from build123d import *

# Parameters (mm, degrees)
ESTRUSIONE_ESTRUSIONE1_DEPTH = 10
FORI_FILETTATI_5_0MM1_D      = 5
FORI_FILETTATI_5_0MM1_DEPTH  = 10
FORI_FILETTATI_5_0MM1_TIP    = 1.502151548
FORI_FILETTATI_5_0MM2_D      = 5
FORI_FILETTATI_5_0MM2_DEPTH  = 10
FORI_FILETTATI_5_0MM2_TIP    = 1.502151548


with BuildPart() as part:
    # Schizzo2 → Estrusione-Estrusione1 (new body)
    with BuildSketch(Plane(origin=(0, 0, 0), x_dir=(0, 0, -1), z_dir=(1, 0, 0))):
        with BuildLine():
            Line((-28, -7), (-9, -7))
            Line((-9, -7), (-9, 0))
            ThreePointArc((-9, 0), (0, 9), (9, 0))
            Line((9, 0), (9, -7))
            Line((9, -7), (28, -7))
            Line((28, -7), (28, -8))
            Line((28, -8), (8, -8))
            Line((8, -8), (8, 0))
            ThreePointArc((8, 0), (0, 8), (-8, 0))
            Line((-8, 0), (-8, -8))
            Line((-8, -8), (-28, -8))
            Line((-28, -8), (-28, -7))
        make_face()
    extrude(amount=ESTRUSIONE_ESTRUSIONE1_DEPTH)

    # Fori filettati Ø5.0mm1
    with Locations(Plane(origin=(5, -7, -18), x_dir=(0, 0, 1), z_dir=(0, 1, 0))):
        with Locations((0, 0)):
            Hole(FORI_FILETTATI_5_0MM1_D / 2, depth=FORI_FILETTATI_5_0MM1_DEPTH)
            with Locations((0, 0, -(FORI_FILETTATI_5_0MM1_DEPTH + FORI_FILETTATI_5_0MM1_TIP / 2))):  # 118° drill point
                Cone(0, FORI_FILETTATI_5_0MM1_D / 2, FORI_FILETTATI_5_0MM1_TIP, mode=Mode.SUBTRACT)

    # Fori filettati Ø5.0mm2
    with Locations(Plane(origin=(5, -7, 18), x_dir=(0, 0, 1), z_dir=(0, 1, 0))):
        with Locations((0, 0)):
            Hole(FORI_FILETTATI_5_0MM2_D / 2, depth=FORI_FILETTATI_5_0MM2_DEPTH)
            with Locations((0, 0, -(FORI_FILETTATI_5_0MM2_DEPTH + FORI_FILETTATI_5_0MM2_TIP / 2))):  # 118° drill point
                Cone(0, FORI_FILETTATI_5_0MM2_D / 2, FORI_FILETTATI_5_0MM2_TIP, mode=Mode.SUBTRACT)


solid = part.part
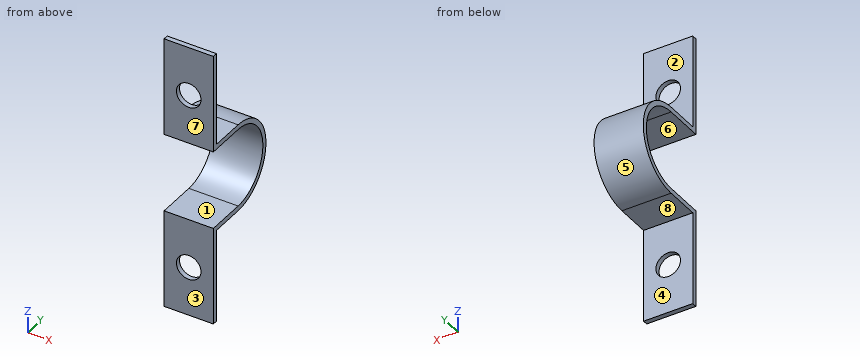
Geometry: final body of the model. Coordinates: model frame, mm. Face numbers are marked on the shaded views. A direction names the side the tool comes from. Coordinates: 2 decimals unless noted, no trailing zeros. Order: outer loops, then holes, each group sorted by start corner. A loop starts at its lowest first (then second) coordinate and runs counter-clockwise, first axis right, second up. Notation, with made-up numbers: M 77.5,86 L 81.5,86 A10 cw 81.5,105 Z; hole C 17,-21.5 d5. An arc over 180 degrees is marked long. One line per question, with ' | ' between items. Start each with the question number.
Item 1: Cut plane D-D, the plane z = 0. Return the cut outline in (x, y), then the cut area to 3 significant figures.
Item 2: Ray query, probe 1 along X at (y, z) = (-7.8, 18); probe 2 along Z at (x, y) = (5.25, -2.25); probe 3 along Y at (x, z) = (3.5, 21). Return the intervals inside material, ascending. Write a range as [from, to].
Item 3: Cut plane A-A, the plane z = 18. Return the cut outline in (x, y).
Item 4: Set-up query: the marked faces 1, 2, 3, 4 and 5. Return all of +Z, -Z, +X, -X, +Y, -Y with unobstructed straight access to the full face (end or side cutting, diameter ignored); none if empty.
Item 5: Cut plane B-B, the plane x = 7. Return the cut outline in (y, z), then the cut area to 3 significant figures.
Item 6: Cut plane C-C, the plane y = 4. Return the cut outline in (x, z).
Item 7: Draft query along Z for the marked faces 6, 7 and 8. Return one class per face: released by +Z, released by -Z, zero draft, split by the parting line, or undercut.
Item 8: Pin query (flat end, axial travel): pin 1 Ø6 at (y, z) = (-5, 14.5) entering from -X; pin 2 Ø2 at (x, y) = (2.5, -3.5) entering from +Z; pin 3 Ø1.5 at (x, z) = (6, 9) entering from +Y; pin 4 Ø5 at (x, z) = (4, 21.5) entering from +Y. Return the tip coordinate at first contact, or that it passes through.
A:
1) outline: M 0,8 L 10,8 L 10,9 L 0,9 Z | area: 10.0 mm2
2) probe 1: x = [0, 2.5], [7.5, 10] | probe 2: z = [-9, -8], [8, 9] | probe 3: y = [-8, -7]
3) outline: M 0,-8 L 2.5,-8 L 2.5,-7 L 0,-7 Z; M 7.5,-8 L 10,-8 L 10,-7 L 7.5,-7 Z
4) face 1: +X, -X, -Y | face 2: +Z, +X, -X, +Y | face 3: +Z, -Z, +X, -X, -Y | face 4: -Z, +X, -X, +Y | face 5: +X, -X, +Y
5) outline: M -8,-28 L -7,-28 L -7,-19.5 L -8,-19.5 Z; M -8,-16.5 L -7,-16.5 L -7,-9 L 0,-9 A9 ccw 0,9 L -7,9 L -7,16.5 L -8,16.5 L -8,8 L 0,8 A8 cw 0,-8 L -8,-8 Z; M -8,19.5 L -7,19.5 L -7,28 L -8,28 Z | area: 74.7 mm2
6) outline: M 0,-8.06 L 10,-8.06 L 10,-6.93 L 0,-6.93 Z; M 0,6.93 L 10,6.93 L 10,8.06 L 0,8.06 Z
7) face 6: undercut | face 7: zero draft | face 8: released by -Z
8) pin 1: stops at x = 0 | pin 2: stops at z = 9 | pin 3: stops at y = 3.6 | pin 4: stops at y = -7
